```python
from build123d import *
from build123d.topology import SkipClean

# Parameters (mm, degrees)
BOSS_EXTRUDE2_DEPTH  = 60
BOSS_EXTRUDE3_START  = 30
SKETCH4_W            = 40
SKETCH4_H            = 10
BOSS_EXTRUDE3_DEPTH  = 20
FILLET1_R            = 10
FILLET2_R            = 10
BOSS_EXTRUDE7_DEPTH  = 10
CUT_EXTRUDE2_DEPTH   = 10
BOSS_EXTRUDE8_START  = -10
BOSS_EXTRUDE8_DEPTH  = 10
BOSS_EXTRUDE18_START = -30
BOSS_EXTRUDE18_DEPTH = 20
MIRROR9_START        = -60
MIRROR9_DEPTH        = 30
BOSS_EXTRUDE20_DEPTH = 5


# Read off the part's stored shape, not the designer's step: Boss-Extrude8, Boss-Extrude18, Mirror9
with BuildPart() as part:
    # Sketch1 → Boss-Extrude2 (new body)
    with BuildSketch(Plane.XY):
        with BuildLine():
            ThreePointArc((40, 0), (0, 40), (-40, 0))
            Line((-40, 0), (-30, 0))
            ThreePointArc((-30, 0), (0, 30), (30, 0))
            Line((30, 0), (40, 0))
        make_face()
    extrude(amount=-BOSS_EXTRUDE2_DEPTH)

    # Sketch4 → Boss-Extrude3 (add)
    with BuildSketch(Plane(origin=(0, 0, 0), x_dir=(0, 0, -1), z_dir=(1, 0, 0)).offset(BOSS_EXTRUDE3_START)):
        with Locations((30, 5)):
            Rectangle(SKETCH4_W, SKETCH4_H)
    boss_extrude3 = extrude(amount=BOSS_EXTRUDE3_DEPTH)

    # Mirror1: Boss-Extrude3 across plane
    add(boss_extrude3.mirror(Plane(origin=(0, 0, 0), x_dir=(0, 0, 1), z_dir=(1, 0, 0))))

    # Fillet1
    fillet1_edges = [part.edges().sort_by_distance(p)[0] for p in [
        (-39.681187851, 5.040171699, -10),
    ]]
    fillet(fillet1_edges, radius=FILLET1_R - 0.0001)  # a hair under: the kernel refuses the full size

    # Fillet2
    fillet2_edges = [part.edges().sort_by_distance(p)[0] for p in [
        (39.681187851, 5.040171699, -10),
    ]]
    fillet(fillet2_edges, radius=FILLET2_R - 0.0001)  # a hair under: the kernel refuses the full size

    # Sketch5 → Boss-Extrude7 (add)
    with BuildSketch(Plane(origin=(0, 10, 0), x_dir=(1, 0, 0), z_dir=(0, 1, 0))):
        with BuildLine():
            ThreePointArc((50, 10), (70, 30), (50, 50))
            Line((50, 50), (50, 38))
            ThreePointArc((50, 38), (55.656854249, 35.656854249), (58, 30))
            ThreePointArc((58, 30), (55.656854249, 24.343145751), (50, 22))
            Line((50, 22), (50, 10))
        make_face()
    boss_extrude7 = extrude(amount=-BOSS_EXTRUDE7_DEPTH)

    # Sketch5<5> → Cut-Extrude2 (cut)
    with SkipClean():  # the faces are left unmerged after this step: merging them gives an invalid solid
        with BuildSketch(Plane(origin=(0, 10, 0), x_dir=(1, 0, 0), z_dir=(0, 1, 0))):
            with BuildLine():
                Line((50, 22), (50, 38))
                ThreePointArc((50, 38), (42, 30), (50, 22))
            make_face()
            with BuildLine():
                ThreePointArc((58, 30), (55.656854249, 35.656854249), (50, 38))
                Line((50, 38), (50, 22))
                ThreePointArc((50, 22), (55.656854249, 24.343145751), (58, 30))
            make_face()
        cut_extrude2 = extrude(amount=-CUT_EXTRUDE2_DEPTH, mode=Mode.SUBTRACT)

    # Mirror3: Boss-Extrude7, Cut-Extrude2 across plane
    with SkipClean():  # the faces are left unmerged after this step: merging them gives an invalid solid
        add(boss_extrude7.mirror(Plane(origin=(0, 0, 0), x_dir=(0, 0, 1), z_dir=(1, 0, 0))))
        add(cut_extrude2.mirror(Plane(origin=(0, 0, 0), x_dir=(0, 0, 1), z_dir=(1, 0, 0))), mode=Mode.SUBTRACT)

    # Boss-Extrude8 outline → Boss-Extrude8 (add)
    with SkipClean():  # the faces are left unmerged after this step: merging them gives an invalid solid
        with BuildSketch(Plane(origin=(0, 0, -60), x_dir=(-1, 0, 0), z_dir=(0, 0, -1)).offset(BOSS_EXTRUDE8_START)):
            with BuildLine():
                ThreePointArc((30.000032068, 99.999679323), (21.213112735, 78.786660512), (0, 69.999967931))
                Line((0, 69.999967931), (0, 85))
                ThreePointArc((0, 85), (-10.606601718, 89.393398282), (-15, 100))
                Line((-15, 100), (-30, 100))
                Line((-30, 100), (-39.207920792, 7.920792079))
                ThreePointArc((-39.207920792, 7.920792079), (0, 40), (39.207920792, 7.920792079))
                Line((39.207920792, 7.920792079), (30.000032068, 99.999679323))
            make_face()
        extrude(amount=BOSS_EXTRUDE8_DEPTH)

    # Boss-Extrude18 outline → Boss-Extrude18 (add)
    with SkipClean():  # the faces are left unmerged after this step: merging them gives an invalid solid
        with BuildSketch(Plane(origin=(0, 0, -60), x_dir=(-1, 0, 0), z_dir=(0, 0, -1)).offset(BOSS_EXTRUDE18_START)):
            with BuildLine():
                ThreePointArc((0, 85), (-10.606601718, 89.393398282), (-15, 100))
                Line((-15, 100), (-30, 100))
                Line((-30, 100), (-30.000032068, 99.999679323))
                ThreePointArc((-30.000032068, 99.999679323), (-21.213112735, 78.786660512), (0, 69.999967931))
                Line((0, 69.999967931), (0, 85))
            make_face()
        extrude(amount=BOSS_EXTRUDE18_DEPTH)

    # Mirror9 outline → Mirror9 (add)
    with SkipClean():  # the faces are left unmerged after this step: merging them gives an invalid solid
        with BuildSketch(Plane.XY.offset(MIRROR9_START)):
            with BuildLine():
                Line((-15, 100), (-30, 100))
                Line((-30, 100), (-30.000032068, 99.999679323))
                ThreePointArc((-30.000032068, 99.999679323), (-21.213112735, 78.786660512), (0, 69.999967931))
                Line((0, 69.999967931), (0, 85))
                ThreePointArc((0, 85), (-10.606601718, 89.393398282), (-15, 100))
            make_face()
        extrude(amount=MIRROR9_DEPTH)

    # Sketch7 → Boss-Extrude20 (add, symmetric)
    with SkipClean():  # the faces are left unmerged after this step: merging them gives an invalid solid
        with BuildSketch(Plane(origin=(0, 0, 0), x_dir=(0, 0, -1), z_dir=(1, 0, 0))):
            Polygon((0, 40), (30, 69.999967931), (30, 70.999967931), (50, 70.999967931), (50, 69.999967931), (50, 40), (50, 39), (0, 39), align=None)
        extrude(amount=BOSS_EXTRUDE20_DEPTH, both=True)


solid = part.part
```
The model under review builds one solid part; all positions refer to its coordinate system, in mm. A direction names the side the tool comes from. Round coordinates to 2 decimals unless told otherwise and drop trailing zeros. Order: outer loops, then holes, each group sorted by start corner. A loop starts at its lowest first (then second) coordinate and runs counter-clockwise, first axis right, second up.
(1) Tool access review of faces 5 (the face through (39.807, 3.925, -54.93)), 6 (the face through (22, 56, -50)), 7 (the face through (-5, 52, -31)): name each direction out of +Z, -Z, +X, -X, +Y, -Y from which nothing blocks a thin tool from reaching the whole face with its end or side.
Working result:
face 5: -Z, +X, +Y
face 6: +Z, +X
face 7: +Z, -X
(2) For P1, Ø15, axis at x = 12.5, y = 91, coming from the +Z side; P2, Ø4, axis at y = 21, z = -39.5, coming from the -X side; P3, Ø0.5, axis at x = 49.5, y = 7.5, coming from the +Z side, all flat-tipped, find the tip position at first contact; note any pin that passes through.
Working result:
P1: stops at z = -30
P2: stops at x = -35.2
P3: stops at z = -10
(3) Take a section at A-A, the plane x = 53.5. State the section outline as (y, z) points.
Working result:
outline: (0, -49.69) - (10, -49.69) - (10, -37.19) - (0, -37.19) - close; (0, -22.81) - (10, -22.81) - (10, -10.31) - (0, -10.31) - close
(4) Wall thickness on L1, parallel to Z at x = 10, y = 71; L2, parallel to Y at x = -51.5, z = -47.5; L3, parallel to X at y = 45, z = -44: over which ranges is each line inside the solid? List them lowest first.
Working result:
L1: z = -60 to -50
L2: y = 0 to 10
L3: x = -5 to 5
(5) Take a section at D-D, the plane x = 0. State the section outline as (y, z) points, plus the area to 3 significant figures.
Working result:
outline: (30, -60) - (85, -60) - (85, -30) - (70, -30) - (40, 0) - (30, 0) - close
area: 2,400 mm2
(6) Mouldability with a two-part tool opening along Y and no side actions: class faces 1 (the face through (-22, 56, -50)), 2 (the face through (0, 85, -45)), 3 (the face through (-44, 5, -50)), 4 (the face through (-23.1, 80.86, -40.14)) as released by +Y, released by -Y, zero draft, split by the parting line, or undercut.
Working result:
face 1: undercut
face 2: released by +Y
face 3: zero draft
face 4: undercut
(7) Take a section at C-C, the plane y = 66.5. State the section outline as (x, z) points, plus the area to 3 significant figures.
Working result:
outline: (-33.35, -60) - (33.35, -60) - (33.35, -50) - (5, -50) - (5, -26.5) - (-5, -26.5) - (-5, -50) - (-33.35, -50) - close
area: 902 mm2
